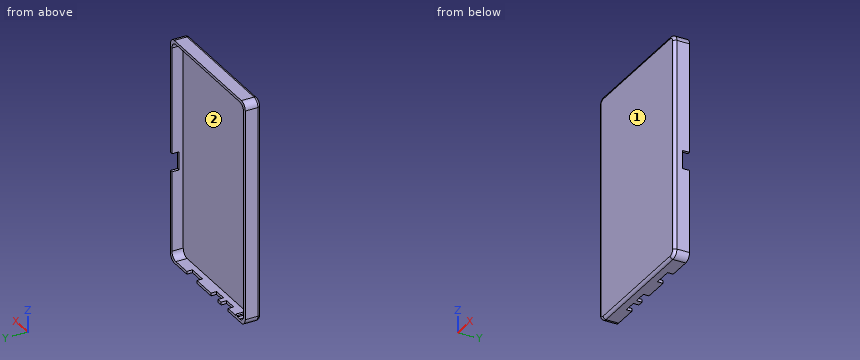
from build123d import *

# Parameters (mm, degrees)
SKETCH_1_W          = 96
SKETCH_1_H          = 160
EXTRUDE_1_DEPTH     = 11
FILLET_1_R          = 5
FILLET_2_R          = 5
FILLET_3_R          = 5
FILLET_4_R          = 5
FILLET_5_R          = 2
CUT_EXTRUDE_1_DEPTH = 8
SKETCH_3_W          = 9
SKETCH_3_H          = 4
SKETCH_3_W_2        = 13
CUT_EXTRUDE_2_DEPTH = 4
SKETCH_4_W          = 13
SKETCH_4_H          = 5
CUT_EXTRUDE_3_DEPTH = 5


with BuildPart() as part:
    # 草图1 → 凸台-拉伸1 (new body)
    with BuildSketch(Plane(origin=(0, 0, 0), x_dir=(1, 0, 0), z_dir=(0, 1, 0))):
        Rectangle(SKETCH_1_W, SKETCH_1_H)
    extrude(amount=EXTRUDE_1_DEPTH)

    # 圆角1
    fillet_1_edges = [part.edges().sort_by_distance(p)[0] for p in [
        (-48, 5.5, -80),
    ]]
    fillet(fillet_1_edges, radius=FILLET_1_R)

    # 圆角2
    fillet_2_edges = [part.edges().sort_by_distance(p)[0] for p in [
        (48, 5.5, -80),
    ]]
    fillet(fillet_2_edges, radius=FILLET_2_R)

    # 圆角3
    fillet_3_edges = [part.edges().sort_by_distance(p)[0] for p in [
        (48, 5.5, 80),
    ]]
    fillet(fillet_3_edges, radius=FILLET_3_R)

    # 圆角4
    fillet_4_edges = [part.edges().sort_by_distance(p)[0] for p in [
        (-48, 5.5, 80),
    ]]
    fillet(fillet_4_edges, radius=FILLET_4_R)

    # 圆角5
    fillet_5_edges = [part.edges().sort_by_distance(p)[0] for p in [
        (-48, 0, 0),
        (-46.535533906, 0, -78.535533906),
        (0, 0, -80),
        (46.535533906, 0, -78.535533906),
        (48, 0, 0),
        (46.535533906, 0, 78.535533906),
        (0, 0, 80),
        (-46.535533906, 0, 78.535533906),
    ]]
    fillet(fillet_5_edges, radius=FILLET_5_R)

    # 草图2 → 切除-拉伸1 (cut)
    with BuildSketch(Plane(origin=(0, 11, 0), x_dir=(1, 0, 0), z_dir=(0, 1, 0))):
        with BuildLine():
            Line((-36, 78), (41, 78))
            ThreePointArc((41, 78), (44.535533906, 76.535533906), (46, 73))
            Line((46, 73), (46, -73))
            ThreePointArc((46, -73), (44.535533906, -76.535533906), (41, -78))
            Line((41, -78), (-41, -78))
            ThreePointArc((-41, -78), (-44.535533906, -76.535533906), (-46, -73))
            Line((-46, -73), (-46, 73))
            ThreePointArc((-46, 73), (-44.535533906, 76.535533906), (-41, 78))
            Line((-41, 78), (-38, 78))
            Line((-38, 78), (-38, 77))
            Line((-38, 77), (-36, 77))
            Line((-36, 77), (-36, 78))
        make_face()
    extrude(amount=-CUT_EXTRUDE_1_DEPTH, mode=Mode.SUBTRACT)

    # 草图3 → 切除-拉伸2 (cut)
    with BuildSketch(Plane.XY.offset(-78)):
        with Locations((-21.5, 9)):
            Rectangle(SKETCH_3_W, SKETCH_3_H)
        with Locations((-8.5, 9)):
            Rectangle(SKETCH_3_W, SKETCH_3_H)
        with Locations((16.277912798, 56.653498761)):
            Rectangle(SKETCH_3_W, SKETCH_3_H)
        with Locations((20.5, 9)):
            Rectangle(SKETCH_3_W_2, SKETCH_3_H)
    extrude(amount=-CUT_EXTRUDE_2_DEPTH, mode=Mode.SUBTRACT)

    # 草图4 → 切除-拉伸3 (cut)
    with BuildSketch(Plane(origin=(48, 0, 0), x_dir=(0, 0, -1), z_dir=(1, 0, 0))):
        with Locations((9.5, 8.5)):
            Rectangle(SKETCH_4_W, SKETCH_4_H)
    extrude(amount=-CUT_EXTRUDE_3_DEPTH, mode=Mode.SUBTRACT)


solid = part.part
Could you check a few things on this model? Use its own coordinates, in mm. Face numbers are marked on the shaded views. Give positions to 0.01 mm unless a question says otherwise; leave off trailing zeros. Order: outer loops, then holes, each group sorted by start corner. A loop starts at its lowest first (then second) coordinate and runs counter-clockwise, first axis right, second up.
Item 1: If we section it at B-B, the plane x = 25: Write out the boundary of the cut face in (y, z).
Item 2: I'm going to push flat-ended pins straight in: pin 1 (0.6 mm diameter, centred on y = 9.5, z = -78.5, fed in from +X); pin 2 (0.6 mm diameter, centred on x = -9.5, z = -78.5, fed in from +Y); pin 3 (0.5 mm diameter, centred on y = 8.5, z = -77.5, fed in from -X). Where does each tip first touch, or does it pass through?
Item 3: If we section it at C-C, the plane z = -22: Write out the boundary of the cut face in (x, y).
Item 4: I need wall thicknesses on line 1 (Z direction, x = 20.5, y = 4.25); line 2 (X direction, y = 3.75, z = -47.5); line 3 (Y direction, x = -32, z = -72.5). Which ranges of each line are inside material? Lowest first, please.
Item 5: If we mould it in two halves opening along Z, with no side actions, what happens to the marked faces 1 and 2? For each: pulls with the +Z half, pulls with the -Z half, needs draft (parallel to the pull), parting line crosses it, or undercut.
Item 6: If we section it at A-A, the plane y = 4.5: Write out the boundary of the cut face in (x, z).
Values:
1. outline: (0, -78) arc R2 ccw to (2, -80) - (7, -80) - (7, -78) - (3, -78) - (3, 78) - (11, 78) - (11, 80) - (2, 80) arc R2 ccw to (0, 78) - close
2. pin 1: stops at x = 46.84
2. pin 2: stops at y = 7
2. pin 3: stops at x = -47.47
3. outline: (-48, 2) arc R2 ccw to (-46, 0) - (46, 0) arc R2 ccw to (48, 2) - (48, 11) - (46, 11) - (46, 3) - (-46, 3) - (-46, 11) - (-48, 11) - close
4. line 1: z = -80 to -78, 78 to 80
4. line 2: x = -48 to -46, 46 to 48
4. line 3: y = 0 to 3
5. face 1: needs draft
5. face 2: undercut
6. outline: (-48, -75) arc R5 ccw to (-43, -80) - (43, -80) arc R5 ccw to (48, -75) - (48, 75) arc R5 ccw to (43, 80) - (-43, 80) arc R5 ccw to (-48, 75) - close; hole (-46, -73) arc R5 ccw to (-41, -78) - (-38, -78) - (-38, -77) - (-36, -77) - (-36, -78) - (41, -78) arc R5 ccw to (46, -73) - (46, 73) arc R5 ccw to (41, 78) - (-41, 78) arc R5 ccw to (-46, 73) - close
